For this review, take the finished solid that the model builds, in its own axes (mm). A direction names the side the tool comes from. Round coordinates to 2 decimals unless told otherwise and drop trailing zeros. Order: outer loops, then holes, each group sorted by start corner. A loop starts at its lowest first (then second) coordinate and runs counter-clockwise, first axis right, second up. Notation, with made-up numbers: M 30,2.25 L 59,2.25 A22 ccw 59,20.25 Z; hole C 47.25,-39.5 d3. An arc over 180 degrees is marked long. Put each result on its own line as item: value.
from build123d import *

# Parameters (mm, degrees)
SKETCH1_R           = 1.5
SKETCH1_W           = 6
SKETCH1_H           = 3
SKETCH1_W_2         = 4
BOSS_EXTRUDE1_DEPTH = 3


with BuildPart() as part:
    # Sketch1 → Boss-Extrude1 (new body)
    with BuildSketch(Plane.XY):
        Polygon((71.188714063, 159.941147496), (74.188714063, 159.941147496), (74.188714063, 162.941147496), (76.320599063, 162.941147496), (76.320599063, 209.041147496), (74.188714063, 209.041147496), (74.188714063, 212.041147496), (71.188714063, 212.041147496), (71.188714063, 209.041147496), (50.952483563, 209.041147496), (50.952483563, 212.041147496), (47.952483563, 212.041147496), (47.952483563, 209.041147496), (45.820598563, 209.041147496), (45.820598563, 162.941147496), (47.952483563, 162.941147496), (47.952483563, 159.941147496), (50.952483563, 159.941147496), (50.952483563, 162.941147496), (71.188714063, 162.941147496), align=None)
        with Locations((61.188714063, 202.541147496)):
            Circle(SKETCH1_R, mode=Mode.SUBTRACT)
        with Locations((61.188714063, 169.441147496)):
            Circle(SKETCH1_R, mode=Mode.SUBTRACT)
        with Locations((52.188714063, 202.541147496)):
            Rectangle(SKETCH1_W, SKETCH1_H, mode=Mode.SUBTRACT)
        with Locations((69.188714063, 202.541147496)):
            Rectangle(SKETCH1_W_2, SKETCH1_H, mode=Mode.SUBTRACT)
        with Locations((52.188714063, 169.441147496)):
            Rectangle(SKETCH1_W, SKETCH1_H, mode=Mode.SUBTRACT)
        with Locations((69.188714063, 169.441147496)):
            Rectangle(SKETCH1_W_2, SKETCH1_H, mode=Mode.SUBTRACT)
    extrude(amount=BOSS_EXTRUDE1_DEPTH)


solid = part.part
(1) To check wall thickness, follow L1, parallel to Y at x = 54, z = 2.8; L2, parallel to X at y = 169.5, z = 2.35; L3, parallel to X at y = 210, z = 2.7. State the ranges of each line that lie inside material, in increasing order.
A:
L1: y = 162.94 to 167.94, 170.94 to 201.04, 204.04 to 209.04
L2: x = 45.82 to 49.19, 55.19 to 59.69, 62.69 to 67.19, 71.19 to 76.32
L3: x = 47.95 to 50.95, 71.19 to 74.19
(2) For faces 4 (the face through (52, 201.041, 1)), 5 (the face through (74.189, 161, 1)), 6 (the face through (47, 162.941, 1)), 7 (the face through (47.952, 211, 1)), list the 3-axis set-ups (+Z, -Z, +X, -X, +Y, -Y) from which the entire face can be reached by the end or side of a thin tool; tool diameter is ignored.
A:
face 4: +Z, -Z
face 5: +Z, -Z, +X, -Y
face 6: +Z, -Z, -X, -Y
face 7: +Z, -Z, -X, +Y
(3) Draft analysis for pull direction Y (two halves, no side actions). For faces 1 (the face through (73, 212.041, 1)), 2 (the face through (52, 167.941, 1)), 3 (the face through (75, 162.941, 1)), state which applies: released by +Y, released by -Y, zero draft, split by the parting line, or undercut.
A:
face 1: released by +Y
face 2: undercut
face 3: released by -Y
(4) Add section C-C on z = 0.95. State how many separate pieces and enclosed holes the cut face has, then the cut area to 3 significant figures.
A:
separate pieces: 1
enclosed holes: 6
area: 1,370 mm2
(5) Add section B-B on y = 170. Give the boundary of the cut face in (x, z), then the cut area to 3 significant figures.
A:
outline: M 45.82,0 L 49.19,0 L 49.19,3 L 45.82,3 Z; M 55.19,0 L 59.8,0 L 59.8,3 L 55.19,3 Z; M 62.58,0 L 67.19,0 L 67.19,3 L 62.58,3 Z; M 71.19,0 L 76.32,0 L 76.32,3 L 71.19,3 Z
area: 53.1 mm2
(6) Add section A-A on x = 68. Give the boundary of the cut face in (y, z).
A:
outline: M 162.94,0 L 167.94,0 L 167.94,3 L 162.94,3 Z; M 170.94,0 L 201.04,0 L 201.04,3 L 170.94,3 Z; M 204.04,0 L 209.04,0 L 209.04,3 L 204.04,3 Z
(7) Add section D-D on x = 57.5. Give the boundary of the cut face in (y, z), then the cut area to 3 significant figures.
A:
outline: M 162.94,0 L 209.04,0 L 209.04,3 L 162.94,3 Z
area: 138 mm2
(8) Insertion check: pin 1 Ø3.5 at (x, y) = (61.19, 169.44) entering from -Z; pin 2 Ø1.5 at (x, z) = (60, 1.5) entering from +Y; pin 3 Ø1.5 at (y, z) = (210.5, 1) entering from -X. Each pin has a flat end and moves straight along its axis. Give the tip position at first contact, or say it passes through.
A:
pin 1: stops at z = 0
pin 2: stops at y = 209.04
pin 3: stops at x = 47.95
